from build123d import *

# Parameters (mm, degrees)
SKETCH002_R     = 6
SKETCH002_R_2   = 3
SKETCH002_R_3   = 1.25
PAD_DEPTH       = 25.4
SKETCH_R        = 13.05
POCKET_DEPTH    = 8
SKETCH003_R     = 13.05
POCKET001_DEPTH = 8
SKETCH004_R     = 5.4
POCKET002_DEPTH = 10


with BuildPart() as part:
    # Sketch002 → Pad (new body)
    with BuildSketch(Plane(origin=(0, 0, 0), x_dir=(1, 0, 0), z_dir=(0, 0, -1))):
        with BuildLine():
            Line((-16.5, 0), (-41.5, 0))
            Line((-41.5, 0), (-41.5, 94.000095))
            ThreePointArc((-41.5, 94.000095), (-42.671573, 96.828522), (-45.499999, 98.000094))
            Line((-54.000002, 98.000094), (-45.499999, 98.000094))
            ThreePointArc((-58, 102.000095), (-56.828428, 99.171668), (-54.000002, 98.000094))
            Line((-58, 153.999905), (-58, 102.000095))
            ThreePointArc((-54.000014, 157.999905), (-56.828432, 156.828327), (-58, 153.999905))
            Line((-54.000014, 157.999905), (-4.000015, 158.000095))
            ThreePointArc((0, 154.000095), (-1.171578, 156.828527), (-4.000015, 158.000095))
            Line((0, 154.000095), (0, 101.999905))
            ThreePointArc((-4.000015, 97.999905), (-1.171578, 99.171473), (0, 101.999905))
            Line((-12.500001, 97.999905), (-4.000015, 97.999905))
            ThreePointArc((-12.500001, 97.999905), (-15.328427, 96.828332), (-16.5, 93.999905))
            Line((-16.5, 93.999905), (-16.5, 0))
        make_face()
        with Locations((-29, 128)):
            Circle(SKETCH002_R, mode=Mode.SUBTRACT)
        with Locations((-29, 64)):
            Circle(SKETCH002_R_2, mode=Mode.SUBTRACT)
        with Locations((-29, 29)):
            Circle(SKETCH002_R_2, mode=Mode.SUBTRACT)
        with Locations((-5.43, 151.57)):
            Circle(SKETCH002_R_3, mode=Mode.SUBTRACT)
        with Locations((-52.57, 151.57)):
            Circle(SKETCH002_R_3, mode=Mode.SUBTRACT)
        with Locations((-52.57, 104.43)):
            Circle(SKETCH002_R_3, mode=Mode.SUBTRACT)
        with Locations((-5.43, 104.43)):
            Circle(SKETCH002_R_3, mode=Mode.SUBTRACT)
    extrude(amount=PAD_DEPTH)

    # Sketch → Pocket (cut)
    with BuildSketch(Plane.XY):
        with Locations((-29, -128)):
            Circle(SKETCH_R)
    extrude(amount=-POCKET_DEPTH, mode=Mode.SUBTRACT)

    # Sketch003 → Pocket001 (cut)
    with BuildSketch(Plane(origin=(0, 0, -25.4), x_dir=(1, 0, 0), z_dir=(0, 0, -1))):
        with Locations((-29, 128)):
            Circle(SKETCH003_R)
    extrude(amount=-POCKET001_DEPTH, mode=Mode.SUBTRACT)

    # Sketch004 → Pocket002 (cut)
    with BuildSketch(Plane.XY):
        with Locations((-29, -29)):
            Circle(SKETCH004_R)
        with Locations((-29, -64)):
            Circle(SKETCH004_R)
    extrude(amount=-POCKET002_DEPTH, mode=Mode.SUBTRACT)


solid = part.part
For this review, take the finished solid that the model builds, in its own axes (mm). A direction names the side the tool comes from. Coordinates: 2 decimals unless noted, no trailing zeros. Order: outer loops, then holes, each group sorted by start corner. A loop starts at its lowest first (then second) coordinate and runs counter-clockwise, first axis right, second up. Notation, with made-up numbers: (6.5, 3.5) -> (64.5, 3.5) arc R29 ccw to (64.5, 29.5) -> close; hole circle Ø11 at (6.5, 89.25). An arc over 180 degrees is marked (long way). Return JSON: item names as keys, results as strings.
1. We need section C-C on z = -14.5. Write out the cut boundary in (x, y), and give its area (3 significant figures).
Answer block:
{"outline": "(-58, -154) arc R4 ccw to (-54, -158) -> (-4, -158) arc R4 ccw to (0, -154) -> (0, -102) arc R4 ccw to (-4, -98) -> (-12.5, -98) arc R4 cw to (-16.5, -94) -> (-16.5, 0) -> (-41.5, 0) -> (-41.5, -94) arc R4 cw to (-45.5, -98) -> (-54, -98) arc R4 ccw to (-58, -102) -> close; hole circle Ø2.5 at (-52.57, -151.57); hole circle Ø2.5 at (-52.57, -104.43); hole circle Ø12 at (-29, -128); hole circle Ø6 at (-29, -64); hole circle Ø6 at (-29, -29); hole circle Ø2.5 at (-5.43, -151.57); hole circle Ø2.5 at (-5.43, -104.43)", "area": "5,730 mm²"}
2. We need section B-B on y = -29. Write out the cut boundary in (x, z).
Answer block:
{"outline": "(-41.5, -25.4) -> (-32, -25.4) -> (-32, -10) -> (-34.4, -10) -> (-34.4, 0) -> (-41.5, 0) -> close; (-26, -25.4) -> (-16.5, -25.4) -> (-16.5, 0) -> (-23.6, 0) -> (-23.6, -10) -> (-26, -10) -> close"}
3. For pin 1 Ø1.5 at (x, y) = (-5.43, -151.57) entering from +Z; pin 2 Ø8 at (x, y) = (-33.5, -127) entering from +Z; pin 3 Ø8 at (x, y) = (-26, -131) entering from -Z; pin 4 Ø1 at (y, z) = (-18, -20.5) entering from -X, all flat-tipped, find the tip position at first contact; note any pin that passes through.
Answer block:
{"pin 1": "through", "pin 2": "z = -8", "pin 3": "z = -17.4", "pin 4": "x = -41.5"}
4. We need section D-D on y = -128. Write out the cut boundary in (x, z).
Answer block:
{"outline": "(-58, -25.4) -> (-42.05, -25.4) -> (-42.05, -17.4) -> (-35, -17.4) -> (-35, -8) -> (-42.05, -8) -> (-42.05, 0) -> (-58, 0) -> close; (-23, -17.4) -> (-15.95, -17.4) -> (-15.95, -25.4) -> (0, -25.4) -> (0, 0) -> (-15.95, 0) -> (-15.95, -8) -> (-23, -8) -> close"}
5. The part is to be moulded in two halves that separate along X. For faces 1 (the flat face through (-8, -98, -13)), 2 (the cylindrical face through (-30.301, -122.143, -12.634)), 3 (the flat face through (-16.5, -48, -13)), 4 (the cylindrical face through (-26.097, -59.447, -4.93)), say which applies: +X half, -X half, draft (parallel to the pull), parting line (faces both ways), or undercut.
Answer block:
{"face 1": "draft", "face 2": "undercut", "face 3": "+X half", "face 4": "undercut"}
6. We need section A-A on x = -29. State how many separate pieces and enclosed holes the cut face has, and give its area (3 significant figures).
Answer block:
{"separate pieces": "4", "enclosed holes": "0", "area": "3,080 mm²"}
7. For line 1 (Y direction, x = -52.57, z = -15); line 2 (Y direction, x = -29, z = -21.5); line 3 (X direction, y = -104.43, z = -17.5), list the stretches that pass through material, from the lowest coordinate up. Write a range as from..to.
Answer block:
{"line 1": "-158..-152.82, -150.32..-105.68, -103.18..-98", "line 2": "-158..-141.05, -114.95..-67, -61..-32, -26..0", "line 3": "-58..-53.82, -51.32..-6.68, -4.18..0"}
8. Machinability: for faces 5 (the cylindrical face through (-26.097, -24.447, -4.93)), 6 (the cylindrical face through (-30.7, -140.94, -21.46)), 7 (the flat face through (-50, -98, -13)), which of the approach directions +Z, -Z, +X, -X, +Y, -Y give a long, thin tool a straight path to every point of the face, cutting with its end or side? Answer none if there is none.
Answer block:
{"face 5": "+Z", "face 6": "-Z", "face 7": "+Z, -Z, -X, +Y"}
